Design review of the part built by this model. Coordinates are the model's own, in mm. Face numbers are marked on the shaded views. A direction names the side the tool comes from. Round coordinates to 2 decimals unless told otherwise and drop trailing zeros. Order: outer loops, then holes, each group sorted by start corner. A loop starts at its lowest first (then second) coordinate and runs counter-clockwise, first axis right, second up. Notation, with made-up numbers: (20.5, 78.5) - (66.5, 78.5) arc R10 ccw to (66.5, 95.5) - close; hole circle Ø7 at (-35, 49.5). An arc over 180 degrees is marked (long way). Write item = value, one per line.
from build123d import *

# Parameters (mm, degrees)
SKETCH_1_W          = 2
SKETCH_1_H          = 18
EXTRUDE_1_DEPTH     = 148
SKETCH_4_W          = 2
SKETCH_4_H          = 8
CUT_EXTRUDE_1_DEPTH = 150.103990557
SKETCH_8_W          = 100
SKETCH_8_H          = 1
EXTRUDE_5_DEPTH     = 10
SKETCH_9_R          = 1.525
CUT_EXTRUDE_3_DEPTH = 150.425566755
SKETCH_10_W         = 12
SKETCH_10_H         = 14
SKETCH_10_W_2       = 91
SKETCH_10_H_2       = 11
CUT_EXTRUDE_4_DEPTH = 150.572724786
FILLET_1_R          = 1
FILLET_2_R          = 1
FILLET_3_R          = 1
FILLET_4_R          = 1
FILLET_5_R          = 1
FILLET_7_R          = 1


with BuildPart() as part:
    # 草图1 → 凸台-拉伸1 (new body)
    with BuildSketch(Plane.XY):
        with Locations((1, 9)):
            Rectangle(SKETCH_1_W, SKETCH_1_H)
    extrude(amount=EXTRUDE_1_DEPTH)

    # 草图4 → 切除-拉伸1 (cut, through all)
    with BuildSketch(Plane(origin=(2, 0, 0), x_dir=(0, 0, -1), z_dir=(1, 0, 0))):
        with Locations((-1, 4)):
            Rectangle(SKETCH_4_W, SKETCH_4_H)
        with Locations((-147, 4)):
            Rectangle(SKETCH_4_W, SKETCH_4_H)
    extrude(amount=-CUT_EXTRUDE_1_DEPTH, mode=Mode.SUBTRACT)

    # 草图8 → 凸台-拉伸5 (add)
    with BuildSketch(Plane.ZY):
        with Locations((74, 17.5)):
            Rectangle(SKETCH_8_W, SKETCH_8_H)
    extrude(amount=EXTRUDE_5_DEPTH)

    # 草图9 → 切除-拉伸3 (cut, through all)
    with BuildSketch(Plane(origin=(0, 18, 0), x_dir=(1, 0, 0), z_dir=(0, 1, 0))):
        with Locations(Location((-4, -30, 0), (0, 0, 270))):
            Circle(SKETCH_9_R)
        with Locations(Location((-4, -118, 0), (0, 0, 270))):
            Circle(SKETCH_9_R)
    extrude(amount=-CUT_EXTRUDE_3_DEPTH, mode=Mode.SUBTRACT)

    # 草图10 → 切除-拉伸4 (cut, through all)
    with BuildSketch(Plane(origin=(2, 0, 0), x_dir=(0, 0, -1), z_dir=(1, 0, 0))):
        with Locations((-15.5, 9)):
            Rectangle(SKETCH_10_W, SKETCH_10_H)
        with Locations((-70, 5.5)):
            Rectangle(SKETCH_10_W_2, SKETCH_10_H_2)
        with Locations((-129.5, 7.5)):
            Rectangle(SKETCH_10_W, SKETCH_10_H_2)
    extrude(amount=-CUT_EXTRUDE_4_DEPTH, mode=Mode.SUBTRACT)

    # 圆角1
    fillet_1_edges = [part.edges().sort_by_distance(p)[0] for p in [
        (-10, 17.5, 24),
        (-10, 17.5, 124),
    ]]
    fillet(fillet_1_edges, radius=FILLET_1_R)

    # 圆角2
    fillet_2_edges = [part.edges().sort_by_distance(p)[0] for p in [
        (1, 11, 115.5),
        (1, 11, 24.5),
    ]]
    fillet(fillet_2_edges, radius=FILLET_2_R)

    # 圆角3
    fillet_3_edges = [part.edges().sort_by_distance(p)[0] for p in [
        (1, 2, 21.5),
        (1, 16, 21.5),
        (1, 16, 9.5),
        (1, 2, 9.5),
    ]]
    fillet(fillet_3_edges, radius=FILLET_3_R)

    # 圆角4
    fillet_4_edges = [part.edges().sort_by_distance(p)[0] for p in [
        (1, 13, 123.5),
        (1, 2, 123.5),
        (1, 2, 135.5),
        (1, 13, 135.5),
    ]]
    fillet(fillet_4_edges, radius=FILLET_4_R)

    # 圆角5
    fillet_5_edges = [part.edges().sort_by_distance(p)[0] for p in [
        (2, 13, 148),
    ]]
    fillet(fillet_5_edges, radius=FILLET_5_R)

    # 圆角7
    fillet_7_edges = [part.edges().sort_by_distance(p)[0] for p in [
        (2, 13, 0),
    ]]
    fillet(fillet_7_edges, radius=FILLET_7_R)


solid = part.part
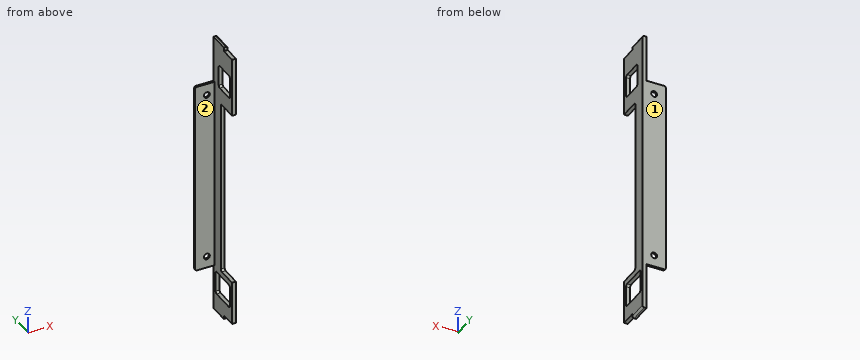
1) For the marked faces 1 and 2, list the 3-axis set-ups (+Z, -Z, +X, -X, +Y, -Y) from which the entire face can be reached by the end or side of a thin tool; tool diameter is ignored.
Findings:
face_1 = +Z, -Z, +X, -X, +Y
face_2 = +Z, -Z, -X, -Y
2) We need section C-C on y = 6.5. Write out the cut boundary in (x, z), and give its area (3 significant figures).
Findings:
outline = (0, 2) - (2, 2) - (2, 9.5) - (0, 9.5) - close; (0, 21.5) - (2, 21.5) - (2, 24.5) - (0, 24.5) - close; (0, 115.5) - (2, 115.5) - (2, 123.5) - (0, 123.5) - close; (0, 135.5) - (2, 135.5) - (2, 146) - (0, 146) - close
area = 58.0 mm^2
3) We need section B-B on x = -4. Write out the cut boundary in (y, z) (3 decimals), and give its area (3 significant figures).
Findings:
outline = (17, 24) - (18, 24) - (18, 28.475) - (17, 28.475) - close; (17, 31.525) - (18, 31.525) - (18, 116.475) - (17, 116.475) - close; (17, 119.525) - (18, 119.525) - (18, 124) - (17, 124) - close
area = 93.9 mm^2
4) To check wall thickness, follow L1, parallel to Y at x = 0.75, z = 19; L2, parallel to Z at x = 1.75, y = 8.5; L3, parallel to X at y = 17.2, z = 30 (3 decimals). State the ranges of each line that lie inside material, in increasing order. Write a range as from..to.
Findings:
L1 = 0..2, 16..18
L2 = 0.34..9.5, 21.5..24.5, 115.5..123.5, 135.5..147.66
L3 = -10..-5.525, -2.475..2
5) Clearance check with flat-ended pins moving along their axes: pin 1 Ø1 at (x, z) = (-8, 103.5) entering from -Y; pin 2 Ø3 at (x, z) = (-3, 15.5) entering from -Y; pin 3 Ø1.6 at (x, y) = (1, 6.5) entering from +Z; pin 4 Ø1 at (x, y) = (1, 5) entering from -Z. State where each tip first meets the part, or that it passes through.
Findings:
pin_1 = 17
pin_2 = through
pin_3 = 146
pin_4 = 2
6) We need section D-D on z = 118. Write out the cut boundary in (x, y) (3 decimals), and give its area (4 significant figures).
Findings:
outline = (-10, 17) - (-5.525, 17) - (-5.525, 18) - (-10, 18) - close; (-2.475, 17) - (0, 17) - (0, 0) - (2, 0) - (2, 18) - (-2.475, 18) - close
area = 42.95 mm^2
7) We need section A-A on z = 30. Write out the cut boundary in (x, y) (3 decimals).
Findings:
outline = (-10, 17) - (-5.525, 17) - (-5.525, 18) - (-10, 18) - close; (-2.475, 17) - (0, 17) - (0, 11) - (2, 11) - (2, 18) - (-2.475, 18) - close
